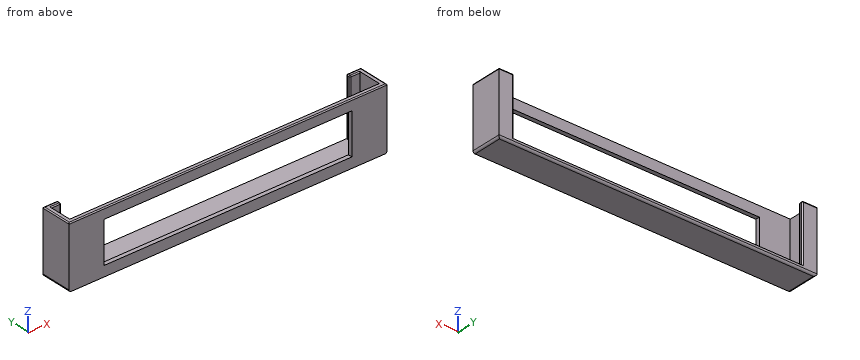
```python
from build123d import *

# Parameters (mm, degrees)
SKETCH_W        = 154
SKETCH_H        = 15
PAD_DEPTH       = 30
SKETCH001_W     = 150
SKETCH001_H     = 11
POCKET_DEPTH    = 28
SKETCH002_W     = 140
SKETCH002_H     = 28
POCKET001_DEPTH = 2
SKETCH003_W     = 120
SKETCH003_H     = 20
POCKET002_DEPTH = 5
FILLET_R        = 0.5
FILLET001_R     = 0.5
FILLET002_R     = 0.5
FILLET003_R     = 1


with BuildPart() as part:
    # Sketch → Pad (new body)
    with BuildSketch(Plane.XY):
        Rectangle(SKETCH_W, SKETCH_H)
    extrude(amount=PAD_DEPTH)

    # Sketch001 → Pocket (cut)
    with BuildSketch(Plane.XY.offset(2)):
        Rectangle(SKETCH001_W, SKETCH001_H)
    extrude(amount=POCKET_DEPTH, mode=Mode.SUBTRACT)

    # Sketch002 (on Face7 of Pocket) → Pocket001 (cut)
    with BuildSketch(Plane.XZ.offset(-7.5)):
        with Locations((0, 16)):
            Rectangle(SKETCH002_W, SKETCH002_H)
    extrude(amount=POCKET001_DEPTH, mode=Mode.SUBTRACT)

    # Sketch003 → Pocket002 (cut)
    with BuildSketch(Plane.XZ.offset(8)):
        with Locations((0, 15)):
            Rectangle(SKETCH003_W, SKETCH003_H)
    extrude(amount=-POCKET002_DEPTH, mode=Mode.SUBTRACT)

    # Fillet
    fillet_edges = [part.edges().sort_by_distance(p)[0] for p in [
        (-70, 7.5, 16),
        (-70, 5.5, 16),
    ]]
    fillet(fillet_edges, radius=FILLET_R)

    # Fillet001
    fillet001_edges = [part.edges().sort_by_distance(p)[0] for p in [
        (70, 5.5, 16),
        (70, 7.5, 16),
    ]]
    fillet(fillet001_edges, radius=FILLET001_R)

    # Fillet002
    fillet002_edges = [part.edges().sort_by_distance(p)[0] for p in [
        (-77, 0, 30),
        (0, -7.5, 30),
        (77, 0, 30),
        (73.75, 7.5, 30),
        (-73.75, 7.5, 30),
    ]]
    fillet(fillet002_edges, radius=FILLET002_R)

    # Fillet003
    fillet003_edges = [part.edges().sort_by_distance(p)[0] for p in [
        (77, 0, 0),
        (0, 7.5, 0),
        (-77, 0, 0),
    ]]
    fillet(fillet003_edges, radius=FILLET003_R)


solid = part.part
```
The listing builds one solid part. Answer for the finished solid, in the listing's coordinates (mm). Round coordinates to 2 decimals unless told otherwise and drop trailing zeros. Order: outer loops, then holes, each group sorted by start corner. A loop starts at its lowest first (then second) coordinate and runs counter-clockwise, first axis right, second up. Notation, with made-up numbers: (-8, 6.5) -> (29, 6.5) arc R21 ccw to (29, 33.5) -> close; hole circle Ø6 at (60, -5.5). An arc over 180 degrees is marked (long way). Answer as CSV lines item,"result".
Q1. A cutting plane is placed at A-A on z = 16.25. Determine the outline of the cut face in (x, y).
Computed values:
outline,"(-77, -7.5) -> (-60, -7.5) -> (-60, -5.5) -> (-75, -5.5) -> (-75, 5.5) -> (-70.5, 5.5) arc R0.5 ccw to (-70, 6) -> (-70, 7) arc R0.5 ccw to (-70.5, 7.5) -> (-77, 7.5) -> close; (60, -7.5) -> (77, -7.5) -> (77, 7.5) -> (70.5, 7.5) arc R0.5 ccw to (70, 7) -> (70, 6) arc R0.5 ccw to (70.5, 5.5) -> (75, 5.5) -> (75, -5.5) -> (60, -5.5) -> close"
Q2. A cutting plane is placed at C-C on y = -2.5. Determine the outline of the cut face in (x, z), plus the area to 3 significant figures.
Computed values:
outline,"(-77, 1) arc R1 ccw to (-76, 0) -> (76, 0) arc R1 ccw to (77, 1) -> (77, 29.5) arc R0.5 ccw to (76.5, 30) -> (75, 30) -> (75, 2) -> (-75, 2) -> (-75, 30) -> (-76.5, 30) arc R0.5 ccw to (-77, 29.5) -> close"
area,"419 mm^2"
Q3. Consider line 1 (Z direction, x = 45, y = -6.25); line 2 (X direction, y = -3.5, z = 12.25); line 3 (X direction, y = 6.5, z = 12.25). Determine where each line is inside the solid, lowest interval first. Write a range as from..to.
Computed values:
line 1,"z = 0..5, 25..30"
line 2,"x = -77..-75, 75..77"
line 3,"x = -77..-70, 70..77"
Q4. Given pin 1 (10 mm diameter, centred on x = -58, z = 11, fed in from +Y); pin 2 (12 mm diameter, centred on x = 7.5, z = 14, fed in from -Y); pin 3 (8 mm diameter, centred on x = 3, y = 1.5, fed in from +Z), each flat-ended and moving along its own axis, determine where each tip first touches the part or whether it passes through.
Computed values:
pin 1,"stops at y = -5.5"
pin 2,"passes through"
pin 3,"stops at z = 2"
Q5. A cutting plane is placed at D-D on x = 68. Determine the outline of the cut face in (y, z), plus the area to 3 significant figures.
Computed values:
outline,"(-7.5, 0) -> (6.5, 0) arc R1 ccw to (7.5, 1) -> (7.5, 2) -> (-5.5, 2) -> (-5.5, 30) -> (-7, 30) arc R0.5 ccw to (-7.5, 29.5) -> close"
area,"85.7 mm^2"
Q6. A cutting plane is placed at B-B on x = -53.5. Determine the outline of the cut face in (y, z).
Computed values:
outline,"(-7.5, 0) -> (6.5, 0) arc R1 ccw to (7.5, 1) -> (7.5, 2) -> (-5.5, 2) -> (-5.5, 5) -> (-7.5, 5) -> close; (-7.5, 25) -> (-5.5, 25) -> (-5.5, 30) -> (-7, 30) arc R0.5 ccw to (-7.5, 29.5) -> close"
